from build123d import *

# Parameters (mm, degrees)
CYLINDER021_R               = 5
CYLINDER021_DEPTH           = 25
CYLINDER022_R               = 5
CYLINDER022_DEPTH           = 15
CYLINDER020_R               = 9
CYLINDER020_DEPTH           = 9.5
BOX007_W                    = 19
BOX007_H                    = 18
BOX007_DEPTH                = 19.5
FILLET_R                    = 8.5
CYLINDER024_R               = 5
CYLINDER024_DEPTH           = 2.5
CYLINDER019_R               = 12
CYLINDER019_DEPTH           = 2.5
CYLINDER027_R               = 8
CYLINDER027_DEPTH           = 12.5
CYLINDER026_R               = 12
CYLINDER026_DEPTH           = 12.5
CYLINDER026_PLACEMENT_ANGLE = 1
FUSION025_PLACEMENT_ANGLE   = 90
FUSION032_PLACEMENT_ANGLE   = 112.48


with BuildPart() as obj1_hole:
    # Cylinder021 → Cylinder021 (new body)
    with BuildSketch(Plane.XY):
        Circle(CYLINDER021_R)
    extrude(amount=CYLINDER021_DEPTH)


with BuildPart() as obj2:
    # Cylinder022 → Cylinder022 (new body)
    with BuildSketch(Plane(origin=(-5, 0, 21), x_dir=(0, 0, -1), z_dir=(1, 0, 0))):
        Circle(CYLINDER022_R)
    extrude(amount=CYLINDER022_DEPTH)

    # Fusion016: union obj1_hole
    add(obj1_hole.part)


with BuildPart() as obj1:
    # Cylinder020 → Cylinder020 (new body)
    with BuildSketch(Plane.XY):
        Circle(CYLINDER020_R)
    extrude(amount=CYLINDER020_DEPTH)


with BuildPart() as obj3:
    # Box007 → Box007 (new body)
    with BuildSketch(Plane(origin=(-9, -9, 9.5), x_dir=(1, 0, 0), z_dir=(0, 0, 1))):
        with Locations((9.5, 9)):
            Rectangle(BOX007_W, BOX007_H)
    extrude(amount=BOX007_DEPTH)

    # Fillet
    fillet_edges = [obj3.edges().sort_by_distance(p)[0] for p in [
        (-9, -9, 19.25),
        (-9, 0, 29),
        (-9, 9, 19.25),
        (0.5, -9, 29),
        (0.5, 9, 29),
    ]]
    fillet(fillet_edges, radius=FILLET_R)

    # Fusion018: union obj1
    add(obj1.part)

    # Cut013: cut obj2
    add(obj2.part, mode=Mode.SUBTRACT)


with BuildPart() as largeplughole:
    # Cylinder024 → Cylinder024 (new body)
    with BuildSketch(Plane.XY):
        Circle(CYLINDER024_R)
    extrude(amount=CYLINDER024_DEPTH)


with BuildPart() as largeplugbase001:
    # Cylinder019 → Cylinder019 (new body)
    with BuildSketch(Plane.XY):
        Circle(CYLINDER019_R)
    extrude(amount=CYLINDER019_DEPTH)

    # Cut008: cut LargePlugHole
    add(largeplughole.part, mode=Mode.SUBTRACT)


with BuildPart() as largeplugwallhole:
    # Cylinder027 → Cylinder027 (new body)
    with BuildSketch(Plane.XY.offset(2.5)):
        Circle(CYLINDER027_R)
    extrude(amount=CYLINDER027_DEPTH)


with BuildPart() as obj4:
    # Cylinder026 → Cylinder026 (new body)
    with BuildSketch(Plane.XY):
        Circle(CYLINDER026_R)
    extrude(amount=CYLINDER026_DEPTH)


with BuildPart() as obj4_1:
    # Cylinder026 placement: moved
    add(obj4.part.moved(Location((0, 0, 2.5))).rotate(Axis((0, 0, 2.5), (0, 0, 1)), CYLINDER026_PLACEMENT_ANGLE))

    # Cut007: cut LargePlugWallHole
    add(largeplugwallhole.part, mode=Mode.SUBTRACT)

    # Fusion025: union LargePlugBase001
    add(largeplugbase001.part)


with BuildPart() as obj4_2:
    # Fusion025 placement: moved
    add(obj4_1.part.moved(Location((10, 0, 21))).rotate(Axis((10, 0, 21), (0, 1, 0)), FUSION025_PLACEMENT_ANGLE))

    # Fusion032: union obj3
    add(obj3.part)


with BuildPart() as obj4_3:
    # Fusion032 placement: moved
    add(obj4_2.part.moved(Location((78, -251.25, 94))).rotate(Axis((78, -251.25, 94), (0, 0, -1)), FUSION032_PLACEMENT_ANGLE))


solid = obj4_3.part
The listing builds one solid part. Answer for the finished solid, in the listing's coordinates (mm). A direction names the side the tool comes from. Coordinates: 2 decimals unless noted, no trailing zeros. Loops run counter-clockwise (first coordinate to the right, second up) from the corner with the lowest first, then second, coordinate; pieces in that order, holes last. Notation, with made-up numbers: M 10,7.25 L 63,7.25 A29 ccw 63,37.25 Z; hole C 60,88.5 d8. An arc over 180 degrees is marked long. Answer in a Markdown table with one row per item.
1) Determine the mould class of faces 5 (the flat face through (81.43, -242.93, 108.92)), 6 (the flat face through (67.254, -257.626, 104.465)), 7 (the cylindrical face through (73.085, -269.413, 107.369)) for opening direction X: released by +X, released by -X, zero draft, split by the parting line, or undercut.
Answers below:
| item | result |
|---|---|
| face 5 | released by +X |
| face 6 | released by -X |
| face 7 | undercut |
2) Given pin 1 (12 mm diameter, centred on x = 84, y = -268, fed in from +Z); pin 2 (6 mm diameter, centred on y = -262, z = 103, fed in from +X); pin 3 (5 mm diameter, centred on y = -247.5, z = 102, fed in from +X), each flat-ended and moving along its own axis, determine where each tip first touches the part or whether it passes through.
Answers below:
| item | result |
|---|---|
| pin 1 | z = 125.42 |
| pin 2 | x = 84.52 |
| pin 3 | x = 87.02 |
3) Find section B-B (z = 101.5). Determine the outline of the cut face in (x, y), then the cut area to 3 significant figures.
Answers below:
| item | result |
|---|---|
| outline | C 78,-251.25 d18; hole C 78,-251.25 d10 |
| area | 176 mm^2 |
4) Find section A-A (z = 113). Determine the outline of the cut face in (x, y).
Answers below:
| item | result |
|---|---|
| outline | M 57.51,-269.83 L 61.28,-271.39 L 66.06,-259.84 L 68.99,-261.05 L 73,-251.35 A5 cw 74.53,-247.65 L 75.68,-244.88 L 84.15,-248.38 L 83,-251.15 A5 cw 81.47,-254.85 L 77.45,-264.55 L 80.38,-265.76 L 75.6,-277.31 L 79.37,-278.87 L 85.11,-265.01 L 82.49,-263.93 L 86.51,-254.23 A8.5 ccw 81.9,-243.13 L 80.98,-242.74 A8.5 ccw 69.88,-247.35 L 65.86,-257.05 L 63.24,-255.97 Z |
5) Which of the six approach directions +Z, -Z, +X, -X, +Y, -Y give full straight-line access (tool end or side, diameter ignored) to faces 1 (the flat face through (81.026, -263.325, 104.465)), 2 (the flat face through (76, -256, 123)), 3 (the flat face through (68.396, -260.804, 115.112)), 4 (the flat face through (75, -260, 103.5))?
Answers below:
| item | result |
|---|---|
| face 1 | -Z, -Y |
| face 2 | +Z, +X, +Y |
| face 3 | none |
| face 4 | -Z |
6) Find the intervals of material crossed by probe 1 along X at (y, z) = (-251.25, 102.5); probe 2 along Z at (x, y) = (71.75, -266); probe 3 along Y at (x, z) = (78, 102.75), in increasing order.
Answers below:
| item | result |
|---|---|
| probe 1 | 69 to 73, 83 to 87 |
| probe 2 | 103 to 107, 123 to 127 |
| probe 3 | -260.25 to -256.25, -246.25 to -242.25 |
